```python
from build123d import *

# Parameters (mm, degrees)
F1_DEPTH       = 3
F3_D           = 7
F3_DEPTH       = 15.24
F3_CSINK_D     = 10
F3_CSINK_ANGLE = 90


with BuildPart() as f1:
    # F0 (on Top) → F1 (new body)
    with BuildSketch(Plane.XY):
        Polygon((32.264434, -25.753669), (32.264434, 0), (32.264434, 26.911139), (0, 26.911139), (-28.502658, 26.911139), (-28.502658, 0), (-28.502658, -25.753669), (0, -25.753669), align=None)
    extrude(amount=F1_DEPTH)

    # F3
    with Locations(Plane.XY.offset(3)):
        with Locations((0, 0)):
            CounterSinkHole(F3_D / 2, F3_CSINK_D / 2, depth=F3_DEPTH, counter_sink_angle=F3_CSINK_ANGLE)


solid = f1.part
```
CAD build for the part. Positions are in the model's coordinates, mm. Round coordinates to 2 decimals unless told otherwise and drop trailing zeros. Write each loop counter-clockwise with the first axis right and the second up, starting at its lowest first coordinate (ties: lowest second). Pieces come first, ordered by that corner, then holes.
Item 1: Mould opens along X. For faces 1 (the flat face through (2, 26.911, 1)), 2 (the cylindrical face through (-3.233, -1.341, 0.74)), 3 (the conical face through (4, 0, 2)), 4 (the flat face through (-28.503, 1, 1)) say: released by +X, released by -X, zero draft, split by the parting line, or undercut.
Filled in:
face 1: zero draft
face 2: undercut
face 3: undercut
face 4: released by -X
Item 2: Band-saw the part on A-A on x = 0. Write the cut outline in (y, z).
Filled in:
outline: (-25.75, 0) - (-3.5, 0) - (-3.5, 1.5) - (-5, 3) - (-25.75, 3) - close; (3.5, 0) - (26.91, 0) - (26.91, 3) - (5, 3) - (3.5, 1.5) - close
Item 3: Drop a flat-ended pin along its axis: pin 1 Ø6.5 at (x, y) = (0, 0) entering from +Z. Give the stop position or say it passes through.
Filled in:
pin 1: passes through
Item 4: Band-saw the part on B-B on y = 0. Write the cut outline in (x, z).
Filled in:
outline: (-28.5, 0) - (-3.5, 0) - (-3.5, 1.5) - (-5, 3) - (-28.5, 3) - close; (3.5, 0) - (32.26, 0) - (32.26, 3) - (5, 3) - (3.5, 1.5) - close
Item 5: Drill centre lines: L1, parallel to Y at x = 0, z = 0.6; L2, parallel to X at y = 0, z = 0.7; L3, parallel to X at y = 1.5, z = 2.2. Where is each one in solid material? Low to high.
Filled in:
L1: y = -25.75 to -3.5, 3.5 to 26.91
L2: x = -28.5 to -3.5, 3.5 to 32.26
L3: x = -28.5 to -3.92, 3.92 to 32.26
